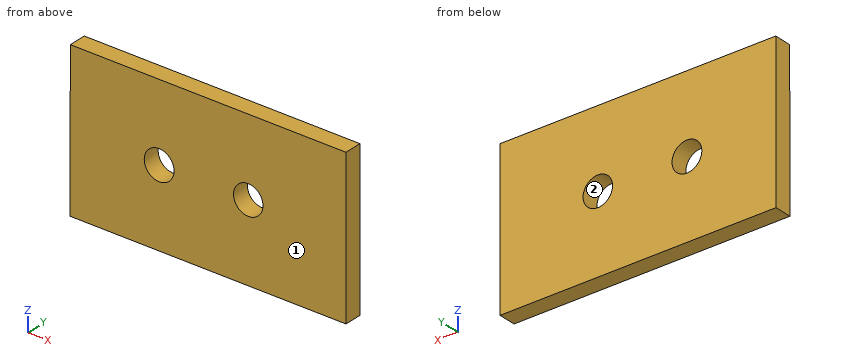
from build123d import *

# Parameters (mm, degrees)
F1_DEPTH = 12.7
F3_D     = 21.59
F5_D     = 21.336


with BuildPart() as f1:
    # F0 (on Front) → F1 (new body)
    with BuildSketch(Plane.XZ):
        Polygon((99.809796, 55.887308), (-99.624716, 55.887308), (-99.808872, -55.887308), (99.809796, -55.887308), align=None)
    extrude(amount=F1_DEPTH)

    # F3 (through all)
    with Locations(Plane.XZ.offset(12.7)):
        with Locations((-35.354935, 0)):
            Hole(F3_D / 2)

    # F5 (through all)
    with Locations(Plane.XZ.offset(12.7)):
        with Locations((29.095007, 0)):
            Hole(F5_D / 2)


solid = f1.part
Can you work these out from the model? Positions are in its coordinate system, mm. Face numbers are marked on the shaded views. Coordinates: 2 decimals unless noted, no trailing zeros. Order: outer loops, then holes, each group sorted by start corner. A loop starts at its lowest first (then second) coordinate and runs counter-clockwise, first axis right, second up. Notation, with made-up numbers: M 39,49 L 91,49 A21 cw 91,71 Z; hole C -27,59.5 d5. An arc over 180 degrees is marked long. Write item = value, one per line.
(1) I need wall thicknesses on line 1 along X through (y, z) = (-8.5, 2.5); line 2 along X through (y, z) = (-11.75, -9); line 3 along X through (y, z) = (-11, -46.5). Which ranges of each line are inside material? Lowest first, please. Write a range as [from, to].
Results are:
line_1 = [-99.71, -45.86], [-24.85, 18.72], [39.47, 99.81]
line_2 = [-99.73, -41.32], [-29.39, 23.37], [34.82, 99.81]
line_3 = [-99.79, 99.81]
(2) For pin 1 Ø19 at (x, z) = (29.1, 0) entering from +Y, with a flat end and sliding along its axis, tell me the tip position at first contact or that it passes through.
Results are:
pin_1 = through
(3) Suppose I cut it at A-A on z = 0. Please give me the cut outline in (x, y), plus the area to 3 significant figures.
Results are:
outline = M -99.72,-12.7 L -46.15,-12.7 L -46.15,0 L -99.72,0 Z; M -24.56,-12.7 L 18.43,-12.7 L 18.43,0 L -24.56,0 Z; M 39.76,-12.7 L 99.81,-12.7 L 99.81,0 L 39.76,0 Z
area = 1,990 mm2
(4) If we mould it in two halves opening along X, with no side actions, what happens to the marked faces 1 and 2? For each: pulls with the +X half, pulls with the -X half, needs draft (parallel to the pull), parting line crosses it, or undercut.
Results are:
face_1 = needs draft
face_2 = undercut
(5) Suppose I cut it at C-C on x = -35.5. Please give me the cut outline in (y, z).
Results are:
outline = M -12.7,-55.89 L 0,-55.89 L 0,-10.79 L -12.7,-10.79 Z; M -12.7,10.79 L 0,10.79 L 0,55.89 L -12.7,55.89 Z
(6) Suppose I cut it at B-B on y = -9.5. Please give me the cut outline in (x, z) (3 decimals), plus the area to 3 significant figures.
Results are:
outline = M -99.809,-55.887 L 99.81,-55.887 L 99.81,55.887 L -99.625,55.887 Z; hole C -35.355,0 d21.59; hole C 29.095,0 d21.336
area = 21,600 mm2
